from build123d import *

# Parameters (mm, degrees)
EXTRUDE_2_DEPTH     = 14.5
SKETCH_2_R          = 3.6
CUT_EXTRUDE_1_DEPTH = 14.5


with BuildPart() as part:
    # 草图1 → 凸台-拉伸2 (new body)
    with BuildSketch(Plane(origin=(0, 0, 0), x_dir=(1, 0, 0), z_dir=(0, 1, 0))):
        with BuildLine():
            ThreePointArc((-13.856406461, -13), (-7.549834433, -17.435595775), (5e-09, -19))
            Line((0, -19), (0, -6))
            ThreePointArc((0, -6), (-6, 0), (0, 6))
            Line((0, 6), (0, 19))
            ThreePointArc((0, 19), (-13.435028843, 13.435028843), (-19, 0))
            ThreePointArc((-19, 0), (-17.667367132, -6.99028888), (-13.856406461, -13))
        make_face()
        with BuildLine():
            Line((0, -6), (0, -19))
            ThreePointArc((5e-09, -19), (7.549834438, -17.435595773), (13.856406461, -13))
            ThreePointArc((13.856406461, -13), (17.667367132, -6.99028888), (19, 0))
            ThreePointArc((19, 0), (13.435028843, 13.435028843), (0, 19))
            Line((0, 19), (0, 6))
            ThreePointArc((0, 6), (4.242640687, 4.242640687), (6, 0))
            ThreePointArc((6, 0), (4.242640687, -4.242640687), (0, -6))
        make_face()
        with BuildLine():
            Line((-19, -13), (-13.856406461, -13))
            ThreePointArc((-13.856406461, -13), (-17.667367132, -6.99028888), (-19, 0))
            Line((-19, 0), (-19, -13))
        make_face()
        with BuildLine():
            ThreePointArc((19, 0), (17.667367132, -6.99028888), (13.856406461, -13))
            Line((13.856406461, -13), (19, -13))
            Line((19, -13), (19, 0))
        make_face()
        with BuildLine():
            Line((5e-09, -19), (35.5, -19))
            Line((35.5, -19), (35.5, -13))
            Line((35.5, -13), (19, -13))
            Line((19, -13), (13.856406461, -13))
            ThreePointArc((13.856406461, -13), (7.549834438, -17.435595773), (5e-09, -19))
        make_face()
        with BuildLine():
            Line((-35.5, -19), (5e-09, -19))
            ThreePointArc((5e-09, -19), (-7.549834433, -17.435595775), (-13.856406461, -13))
            Line((-13.856406461, -13), (-19, -13))
            Line((-19, -13), (-35.5, -13))
            Line((-35.5, -13), (-35.5, -19))
        make_face()
    extrude(amount=EXTRUDE_2_DEPTH)

    # 草图2 → 切除-拉伸1 (cut)
    with BuildSketch(Plane(origin=(0, 0, 13), x_dir=(-1, 0, 0), z_dir=(0, 0, -1))):
        with Locations((-28, 7.25)):
            Circle(SKETCH_2_R)
        with Locations((28, 7.25)):
            Circle(SKETCH_2_R)
    extrude(amount=-CUT_EXTRUDE_1_DEPTH, mode=Mode.SUBTRACT)


solid = part.part
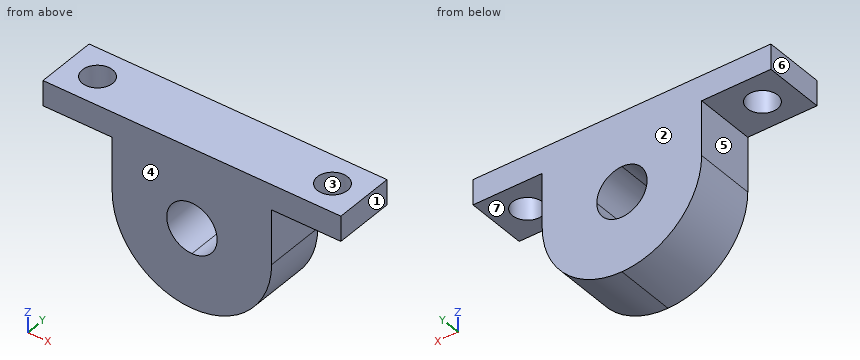
For this review, take the finished solid that the model builds, in its own axes (mm). Face numbers are marked on the shaded views. A direction names the side the tool comes from. Round coordinates to 2 decimals unless told otherwise and drop trailing zeros. Write each loop counter-clockwise with the first axis right and the second up, starting at its lowest first coordinate (ties: lowest second). Pieces come first, ordered by that corner, then holes. Notation, with made-up numbers: (59, -1) -> (70, -1) arc R23 ccw to (70, 29) -> close; hole circle Ø11 at (54.5, -33). An arc over 180 degrees is marked (long way). Use CSV: the item, a comma, the result in double quotes.
(1) Consider section B-B, the plane x = -28. Give the boundary of the cut face in (y, z).
Computed values:
outline,"(0, 13) -> (3.65, 13) -> (3.65, 19) -> (0, 19) -> close; (10.85, 13) -> (14.5, 13) -> (14.5, 19) -> (10.85, 19) -> close"
(2) Clearance check with flat-ended pins moving along their axes: P1, Ø1.5, axis at x = 28.5, y = 1.5, coming from the -Z side; P2, Ø6.5, axis at x = -28, y = 7.25, coming from the +Z side; P3, Ø5, axis at x = -10.5, z = -5, coming from the -Y side; P4, Ø4, axis at y = 4.5, z = 0.5, coming from the +X side. State where each tip first meets the part, or that it passes through.
Computed values:
P1,"z = 13"
P2,"through"
P3,"y = 0"
P4,"x = 19"
(3) Consider section D-D, the plane y = 12.75. Give the boundary of the cut face in (x, z).
Computed values:
outline,"(-35.5, 13) -> (-19, 13) -> (-19, 0) arc R19 ccw to (19, 0) -> (19, 13) -> (35.5, 13) -> (35.5, 19) -> (-35.5, 19) -> close; hole circle Ø12 at (0, 0)"
(4) Consider section C-C, the plane z = -4.5. Give the boundary of the cut face in (x, y), plus the area to 3 significant figures.
Computed values:
outline,"(-18.46, 0) -> (-3.97, 0) -> (-3.97, 14.5) -> (-18.46, 14.5) -> close; (3.97, 0) -> (18.46, 0) -> (18.46, 14.5) -> (3.97, 14.5) -> close"
area,"420 mm²"
(5) Draft analysis for pull direction Y (two halves, no side actions). For the marked faces 1, 2, 3 and 4, state which applies: +Y half, -Y half, draft (parallel to the pull), parting line (faces both ways), or undercut.
Computed values:
face 1,"draft"
face 2,"+Y half"
face 3,"undercut"
face 4,"-Y half"
(6) To check wall thickness, follow L1, parallel to Y at x = -28, z = 17; L2, parallel to X at y = 6.75, z = 3.5; L3, parallel to Z at x = -25, y = 12.75. State the ranges of each line that lie inside material, in increasing order. Write a range as [from, to].
Computed values:
L1,"[0, 3.65], [10.85, 14.5]"
L2,"[-19, -4.87], [4.87, 19]"
L3,"[13, 19]"
(7) For the marked faces 5, 6 and 7, list the 3-axis set-ups (+Z, -Z, +X, -X, +Y, -Y) from which the entire face can be reached by the end or side of a thin tool; tool diameter is ignored.
Computed values:
face 5,"-Z, -X, +Y, -Y"
face 6,"+Z, -Z, -X, +Y, -Y"
face 7,"-Z, +X, +Y, -Y"
(8) Consider section A-A, the plane y = 7.25. Give the boundary of the cut face in (x, z).
Computed values:
outline,"(-35.5, 13) -> (-31.6, 13) -> (-31.6, 19) -> (-35.5, 19) -> close; (-24.4, 13) -> (-19, 13) -> (-19, 0) arc R19 ccw to (19, 0) -> (19, 13) -> (24.4, 13) -> (24.4, 19) -> (-24.4, 19) -> close; (31.6, 13) -> (35.5, 13) -> (35.5, 19) -> (31.6, 19) -> close; hole circle Ø12 at (0, 0)"
